For this review, take the finished solid that the model builds, in its own axes (mm). A direction names the side the tool comes from. Round coordinates to 2 decimals unless told otherwise and drop trailing zeros. Loops run counter-clockwise (first coordinate to the right, second up) from the corner with the lowest first, then second, coordinate; pieces in that order, holes last.
1. Clearance check with flat-ended pins moving along their axes: pin 1 Ø1.6 at (x, z) = (14, 1.5) entering from +Y; pin 2 Ø25 at (x, y) = (-19, -9.5) entering from +Z; pin 3 Ø2 at (x, z) = (-13.5, 1.5) entering from -Y. State where each tip first meets the part, or that it passes through.
2. Tool access review of faces 1 (the flat face through (-1, -44, -20)), 2 (the flat face through (0, 40, -16)): name each direction out of +Z, -Z, +X, -X, +Y, -Y from which nothing blocks a thin tool from reaching the whole face with its end or side.
3. Consider section A-A on z = -2. State the section outline as (x, y) points, then the cut area to 3 significant figures.
4. To check wall thickness, follow line 1 along X through (y, z) = (-17.5, -9); line 2 along Y through (x, z) = (-36.5, -12). State the ranges of each line that lie inside material, in increasing order.
5. Draft analysis for pull direction X (two halves, no side actions). For faces 3 (the cylindrical face through (0.55, -43.4, 1.43)), 4 (the flat face through (-44, 1, -20)), 5 (the flat face through (40, 0, -16)), 6 (the cylindrical face through (43.4, 0.55, 1.43)), state which applies: released by +X, released by -X, zero draft, split by the parting line, or undercut.
from build123d import *

# Parameters (mm, degrees)
F1_DEPTH = 40
F2_DEPTH = 38
F3_DEPTH = 2
F4_R     = 1.99999
F5_R     = 5


# Not quite as in the source:
# - a fillet or chamfer is up to 0.001 mm smaller than in the source, because OpenCascade refuses the exact size


with BuildPart() as f1:
    # F0 (on Top) → F1 (new body)
    with BuildSketch(Plane.XY):
        with BuildLine():
            Line((-39, -44), (39, -44))
            ThreePointArc((39, -44), (42.5355339059, -42.5355339059), (44, -39))
            Line((44, -39), (44, 39))
            ThreePointArc((44, 39), (42.5355339059, 42.5355339059), (39, 44))
            Line((39, 44), (-39, 44))
            ThreePointArc((-39, 44), (-42.5355339059, 42.5355339059), (-44, 39))
            Line((-44, 39), (-44, -39))
            ThreePointArc((-44, -39), (-42.5355339059, -42.5355339059), (-39, -44))
        make_face()
        Polygon((42, -36.3431457505), (42, -42), (36.3431457505, -42), (-36.3431457505, -42), (-42, -42), (-42, -36.3431457505), (-42, 36.3431457505), (-42, 42), (-36.3431457505, 42), (36.3431457505, 42), (42, 42), (42, 36.3431457505), align=None, mode=Mode.SUBTRACT)
        Polygon((-35.5147186258, -40), (35.5147186258, -40), (40, -35.5147186258), (40, 35.5147186258), (35.5147186258, 40), (-35.5147186258, 40), (-40, 35.5147186258), (-40, -35.5147186258), align=None)
        Polygon((40, 35.5147186258), (40, 38.3431457505), (38.3431457505, 40), (35.5147186258, 40), align=None)
        Polygon((40, 38.3431457505), (42, 36.3431457505), (42, 42), (36.3431457505, 42), (38.3431457505, 40), (40, 40), align=None)
        Polygon((38.3431457505, 40), (40, 38.3431457505), (40, 40), align=None)
        Polygon((40, -38.3431457505), (42, -36.3431457505), (42, 36.3431457505), (40, 38.3431457505), (40, 35.5147186258), (40, -35.5147186258), align=None)
        Polygon((38.3431457505, 40), (36.3431457505, 42), (-36.3431457505, 42), (-38.3431457505, 40), (-35.5147186258, 40), (35.5147186258, 40), align=None)
        Polygon((-38.3431457505, 40), (-40, 38.3431457505), (-40, 35.5147186258), (-35.5147186258, 40), align=None)
        Polygon((-40, 40), (-40, 38.3431457505), (-38.3431457505, 40), align=None)
        Polygon((-42, 42), (-42, 36.3431457505), (-40, 38.3431457505), (-40, 40), (-38.3431457505, 40), (-36.3431457505, 42), align=None)
        Polygon((-42, 36.3431457505), (-42, -36.3431457505), (-40, -38.3431457505), (-40, -35.5147186258), (-40, 35.5147186258), (-40, 38.3431457505), align=None)
        Polygon((-40, -38.3431457505), (-38.3431457505, -40), (-35.5147186258, -40), (-40, -35.5147186258), align=None)
        Polygon((-40, -40), (-38.3431457505, -40), (-40, -38.3431457505), align=None)
        Polygon((-42, -42), (-36.3431457505, -42), (-38.3431457505, -40), (-40, -40), (-40, -38.3431457505), (-42, -36.3431457505), align=None)
        Polygon((-36.3431457505, -42), (36.3431457505, -42), (38.3431457505, -40), (35.5147186258, -40), (-35.5147186258, -40), (-38.3431457505, -40), align=None)
        Polygon((35.5147186258, -40), (38.3431457505, -40), (40, -38.3431457505), (40, -35.5147186258), align=None)
        Polygon((40, -38.3431457505), (38.3431457505, -40), (40, -40), align=None)
        Polygon((36.3431457505, -42), (42, -42), (42, -36.3431457505), (40, -38.3431457505), (40, -40), (38.3431457505, -40), align=None)
    extrude(amount=-F1_DEPTH)

    # F0 (on Top) → F2 (cut)
    with BuildSketch(Plane.XY):
        Polygon((-35.5147186258, -40), (35.5147186258, -40), (40, -35.5147186258), (40, 35.5147186258), (35.5147186258, 40), (-35.5147186258, 40), (-40, 35.5147186258), (-40, -35.5147186258), align=None)
    extrude(amount=-F2_DEPTH, mode=Mode.SUBTRACT)

    # F0 (on Top) → F3 (join)
    with BuildSketch(Plane.XY):
        with BuildLine():
            Line((-39, -44), (39, -44))
            ThreePointArc((39, -44), (42.5355339059, -42.5355339059), (44, -39))
            Line((44, -39), (44, 39))
            ThreePointArc((44, 39), (42.5355339059, 42.5355339059), (39, 44))
            Line((39, 44), (-39, 44))
            ThreePointArc((-39, 44), (-42.5355339059, 42.5355339059), (-44, 39))
            Line((-44, 39), (-44, -39))
            ThreePointArc((-44, -39), (-42.5355339059, -42.5355339059), (-39, -44))
        make_face()
        Polygon((42, -36.3431457505), (42, -42), (36.3431457505, -42), (-36.3431457505, -42), (-42, -42), (-42, -36.3431457505), (-42, 36.3431457505), (-42, 42), (-36.3431457505, 42), (36.3431457505, 42), (42, 42), (42, 36.3431457505), align=None, mode=Mode.SUBTRACT)
        Polygon((-42, 42), (-42, 36.3431457505), (-40, 38.3431457505), (-40, 40), (-38.3431457505, 40), (-36.3431457505, 42), align=None)
        Polygon((-40, 40), (-40, 38.3431457505), (-38.3431457505, 40), align=None)
        Polygon((40, 38.3431457505), (42, 36.3431457505), (42, 42), (36.3431457505, 42), (38.3431457505, 40), (40, 40), align=None)
        Polygon((38.3431457505, 40), (40, 38.3431457505), (40, 40), align=None)
        Polygon((36.3431457505, -42), (42, -42), (42, -36.3431457505), (40, -38.3431457505), (40, -40), (38.3431457505, -40), align=None)
        Polygon((40, -38.3431457505), (38.3431457505, -40), (40, -40), align=None)
        Polygon((-42, -42), (-36.3431457505, -42), (-38.3431457505, -40), (-40, -40), (-40, -38.3431457505), (-42, -36.3431457505), align=None)
        Polygon((-40, -40), (-38.3431457505, -40), (-40, -38.3431457505), align=None)
    extrude(amount=F3_DEPTH)

    # F4 (radius 2 in the source; OpenCascade refuses exactly that, so slightly less here)
    f4_edges = [f1.edges().sort_by_distance(p)[0] for p in [
        (-42.535534, -42.535534, 2),
    ]]
    fillet(f4_edges, radius=F4_R)

    # F5
    f5_edges = [f1.edges().sort_by_distance(p)[0] for p in [
        (0, 40, -38),
        (-40, 0, -38),
        (-37.757359, 37.757359, -38),
        (-37.757359, -37.757359, -38),
        (0, -40, -38),
        (37.757359, -37.757359, -38),
        (40, 0, -38),
        (37.757359, 37.757359, -38),
    ]]
    fillet(f5_edges, radius=F5_R)


solid = f1.part
Resolved:
1. pin 1: stops at y = 43.87
1. pin 2: stops at z = -38
1. pin 3: stops at y = -43.94
2. face 1: +Z, -Z, +X, -X, -Y
2. face 2: +Z
3. outline: (-44, -39) arc R5 ccw to (-39, -44) - (39, -44) arc R5 ccw to (44, -39) - (44, 39) arc R5 ccw to (39, 44) - (-39, 44) arc R5 ccw to (-44, 39) - close; hole (-40, -35.51) - (-35.51, -40) - (35.51, -40) - (40, -35.51) - (40, 35.51) - (35.51, 40) - (-35.51, 40) - (-40, 35.51) - close
3. area: 1,360 mm2
4. line 1: x = -44 to -40, 40 to 44
4. line 2: y = -44 to -39.01, 39.01 to 44
5. face 3: zero draft
5. face 4: released by -X
5. face 5: undercut
5. face 6: released by +X
